Drawing for the job (mm, zero at the part's lowest x, y, z). A direction names the side the tool comes from. Round coordinates to 2 decimals unless told otherwise and drop trailing zeros. Order: outer loops, then holes, each group sorted by start corner. A loop starts at its lowest first (then second) coordinate and runs counter-clockwise, first axis right, second up. Notation, with made-up numbers: M 77,67.5 L 118,67.5 A18 cw 118,75.5 Z; hole C 75,37 d9. An arc over 180 degrees is marked long. Answer as CSV lines item,"result". Start each with the question number.
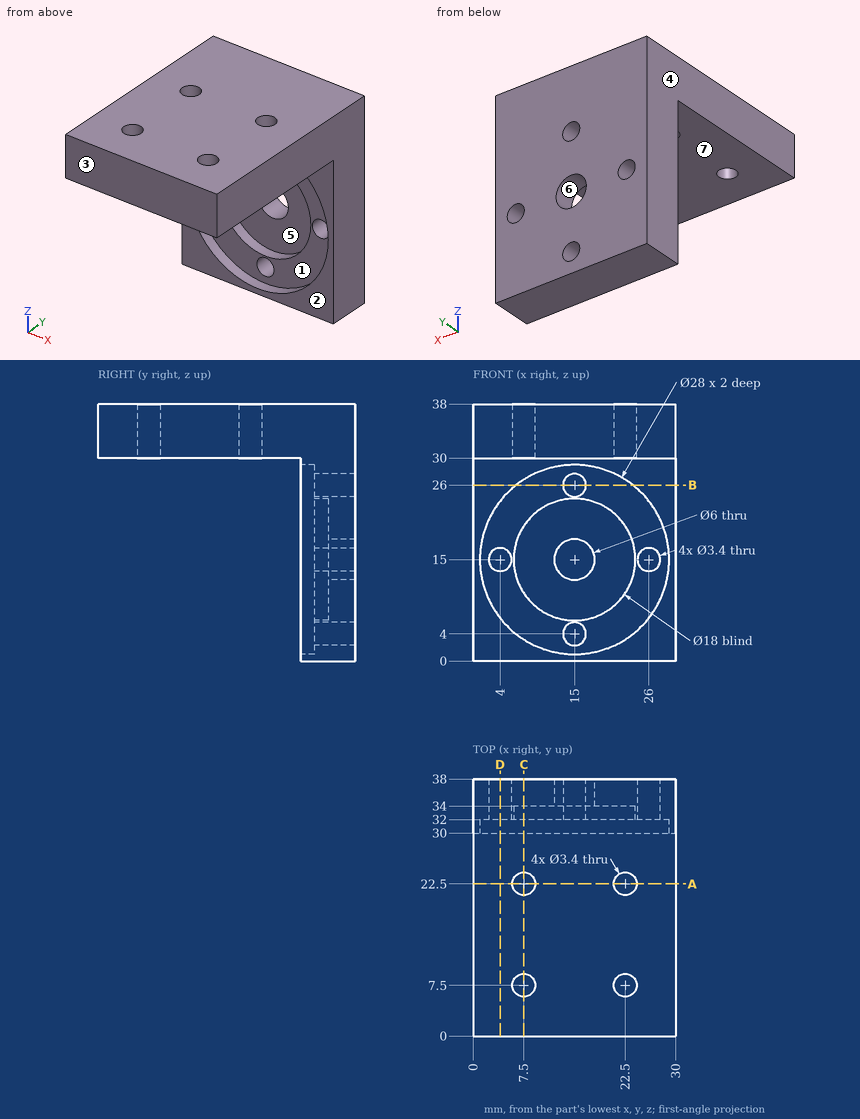
Q1. Tool access for the marked faces 1, 2 and 3: list every direction of +Z, -Z, +X, -X, +Y, -Y with a clear straight run to the whole face (end or side of a thin tool).
Q2. Probe line 1 along Y through (x, z) = (22.5, 35.75); line 2 along X through (y, z) = (7.5, 32.25); line 3 along Y through (x, z) = (21.75, 30.5). List the from-to ranges inside material, lowest first. Write a range as from..to.
Q3. Band-saw the part on B-B, the plane z = 26. Write the cut outline in (x, y), then the cut area to 3 significant figures.
Q4. Band-saw the part on C-C, the plane x = 7.5. Write the cut outline in (y, z).
Q5. Drop flat-ended pins along their axis: P1, Ø4, axis at x = 7.5, y = 22.5, coming from the +Z side; P2, Ø3, axis at x = 15, z = 26, coming from the -Y side (3 decimals); P3, Ø15, axis at x = 11.5, z = 11, coming from the -Y side; P4, Ø6, axis at x = 4.5, y = 16, coming from the -Z side. Give the stop position or say it passes through.
Q6. Mould opens along Z. For the marked faces 4, 5, 6 and 7 say: +Z half, -Z half, draft (parallel to the pull), parting line (faces both ways), or undercut.
Q7. Band-saw the part on D-D, the plane x = 4. Write the cut outline in (y, z).
Q8. Band-saw the part on A-A, the plane y = 22.5. Write the cut outline in (x, z).
Answer:
1,face 1,"-Y"
1,face 2,"-Z, +X, -X, -Y"
1,face 3,"+Z, -Z, +X, -X, -Y"
2,line 1,"y = 0..5.8, 9.2..20.8, 24.2..38"
2,line 2,"x = 0..5.8, 9.2..20.8, 24.2..30"
2,line 3,"y = 0..5.97, 9.03..20.97, 24.03..38"
3,outline,"M 0,30 L 6.34,30 L 6.34,32 L 13.3,32 L 13.3,38 L 0,38 Z; M 16.7,32 L 23.66,32 L 23.66,30 L 30,30 L 30,38 L 16.7,38 Z"
3,area,"185 mm^2"
4,outline,"M 0,30 L 5.8,30 L 5.8,38 L 0,38 Z; M 9.2,30 L 20.8,30 L 20.8,38 L 9.2,38 Z; M 24.2,30 L 30,30 L 30,26.82 L 32,26.82 L 32,19.97 L 34,19.97 L 34,10.03 L 32,10.03 L 32,3.18 L 30,3.18 L 30,0 L 38,0 L 38,38 L 24.2,38 Z"
5,P1,"stops at z = 38"
5,P2,"passes through"
5,P3,"stops at y = 32"
5,P4,"stops at z = 30"
6,face 4,"draft"
6,face 5,"undercut"
6,face 6,"undercut"
6,face 7,"-Z half"
7,outline,"M 0,30 L 30,30 L 30,23.66 L 32,23.66 L 32,16.7 L 38,16.7 L 38,38 L 0,38 Z; M 30,0 L 38,0 L 38,13.3 L 32,13.3 L 32,6.34 L 30,6.34 Z"
8,outline,"M 0,30 L 5.8,30 L 5.8,38 L 0,38 Z; M 9.2,30 L 20.8,30 L 20.8,38 L 9.2,38 Z; M 24.2,30 L 30,30 L 30,38 L 24.2,38 Z"
